The model under review builds one solid part; all positions refer to its coordinate system, in mm. A direction names the side the tool comes from. Give positions to 0.01 mm unless a question says otherwise; leave off trailing zeros. Loops run counter-clockwise (first coordinate to the right, second up) from the corner with the lowest first, then second, coordinate; pieces in that order, holes last. Notation, with made-up numbers: (1.5, 32) - (45.5, 32) arc R26 ccw to (45.5, 65) - close; hole circle Ø6 at (21.25, 42). An arc over 180 degrees is marked (long way). Return JSON: item names as keys, results as strings. Group by question number.
from build123d import *

# Parameters (mm, degrees)
F0_W         = 2.75
F0_H         = 20
F1_DEPTH     = 16
F2_W         = 5.15
F2_H         = 10.3
F3_DEPTH     = 2.75
F4_DEPTH     = 15
F5_T1_DEPTH  = 13.2999992773
F5_T3_DEPTH  = 13.2999992773
F5_T9_DEPTH  = 21.6634917276
F5_T14_DEPTH = 25.0997612432
F5_T22_DEPTH = 21.6634917276
F5_T27_DEPTH = 25.0997612432
F5_T35_DEPTH = 22.0158699277
F5_T40_DEPTH = 25.0997612432
F5_T48_DEPTH = 25.0997612432
F5_T53_DEPTH = 22.0158699277
F6_R         = 5


# Not quite as in the source:
# - a fillet or chamfer that OpenCascade refuses, or shapes differently, is made with other operations: its cross-section is extruded or revolved along the edge and cut away or added
# - a feature names something its author has since deleted; it is built from what else it names


with BuildPart() as f1:
    # F0 (on Top) → F1 (new body)
    with BuildSketch(Plane.XY):
        Rectangle(F0_W, F0_H)
    extrude(amount=F1_DEPTH)

    # F2 (on face) → F3 (join)
    with BuildSketch(Plane.YZ.offset(1.375)):
        Polygon((0, 16), (-10, 16), (-10, 0), (0, 0), (0, 1.4159553841), (-6.6499996386, 1.4159553841), (-6.6499996386, 14.7159546614), (0, 14.7159546614), align=None)
        Polygon((10, 16), (0, 16), (0, 14.7159546614), (6.6499996386, 14.7159546614), (6.6499996386, 1.4159553841), (0, 1.4159553841), (0, 0), (10, 0), align=None)
        with Locations((-2.575, 8.0659550227)):
            Rectangle(F2_W, F2_H)
        with Locations((2.575, 8.0659550227)):
            Rectangle(F2_W, F2_H)
        Polygon((0, 13.2159550227), (0, 14.7159546614), (-6.6499996386, 14.7159546614), (-6.6499996386, 1.4159553841), (0, 1.4159553841), (0, 2.9159550227), (-5.15, 2.9159550227), (-5.15, 13.2159550227), align=None)
        Polygon((6.6499996386, 14.7159546614), (0, 14.7159546614), (0, 13.2159550227), (5.15, 13.2159550227), (5.15, 2.9159550227), (0, 2.9159550227), (0, 1.4159553841), (6.6499996386, 1.4159553841), align=None)
    extrude(amount=-F3_DEPTH)

    # F2 (on face) → F4 (join)
    with BuildSketch(Plane.YZ.offset(1.375)):
        Polygon((0, 13.2159550227), (0, 14.7159546614), (-6.6499996386, 14.7159546614), (-6.6499996386, 1.4159553841), (0, 1.4159553841), (0, 2.9159550227), (-5.15, 2.9159550227), (-5.15, 13.2159550227), align=None)
        Polygon((6.6499996386, 14.7159546614), (0, 14.7159546614), (0, 13.2159550227), (5.15, 13.2159550227), (5.15, 2.9159550227), (0, 2.9159550227), (0, 1.4159553841), (6.6499996386, 1.4159553841), align=None)
    extrude(amount=F4_DEPTH)

    # F5: fillet of radius 5 on 6 edges, made by hand

    # F5_s2 → F5_t1 (join)
    with BuildSketch(Plane.XZ.offset(-6.6499996386)):
        with BuildLine():
            ThreePointArc((1.375, 16), (2.9287180617, 15.0479907955), (4.7203969801, 14.7159546614))
            Line((4.7203969801, 14.7159546614), (1.375, 14.7159546614))
            Line((1.375, 14.7159546614), (1.375, 16))
        make_face()
        with BuildLine():
            ThreePointArc((1.375, 0), (2.9798891295, 1.0484613517), (4.8613482602, 1.4159553841))
            Line((4.8613482602, 1.4159553841), (1.375, 1.4159553841))
            Line((1.375, 1.4159553841), (1.375, 0))
        make_face()
    extrude(amount=F5_T1_DEPTH)

    # F5_s4 → F5_t3 (join)
    with BuildSketch(Plane.XY.offset(1.4159553841)):
        with BuildLine():
            ThreePointArc((1.375, -10), (3.2009454046, -7.5726231419), (6.0949047864, -6.6499996386))
            Line((6.0949047864, -6.6499996386), (1.375, -6.6499996386))
            Line((1.375, -6.6499996386), (1.375, -10))
        make_face()
        with BuildLine():
            ThreePointArc((1.375, 10), (3.2009454046, 7.5726231419), (6.0949047864, 6.6499996386))
            Line((6.0949047864, 6.6499996386), (1.375, 6.6499996386))
            Line((1.375, 6.6499996386), (1.375, 10))
        make_face()
    extrude(amount=F5_T3_DEPTH)


with BuildPart() as f5_tool7:
    # F5_s8 → F5_t9 (new body)
    with BuildSketch(Plane.XZ.offset(-15.013492089)):
        with BuildLine():
            ThreePointArc((1.375, 16), (2.9287180617, 15.0479907955), (4.7203969801, 14.7159546614))
            Line((4.7203969801, 14.7159546614), (1.375, 14.7159546614))
            Line((1.375, 14.7159546614), (1.375, 16))
        make_face()
    extrude(amount=F5_T9_DEPTH)

    split(bisect_by=Plane.XZ.offset(-10), keep=Keep.TOP)

    split(bisect_by=Plane.XZ.offset(-6.6499996386), keep=Keep.BOTTOM)


with BuildPart() as f5_tool12:
    # F5_s13 → F5_t14 (new body)
    with BuildSketch(Plane.XY.offset(1.4159553841)):
        with BuildLine():
            ThreePointArc((1.375, 10), (3.2009454046, 7.5726231419), (6.0949047864, 6.6499996386))
            Line((6.0949047864, 6.6499996386), (1.375, 6.6499996386))
            Line((1.375, 6.6499996386), (1.375, 10))
        make_face()
    extrude(amount=F5_T14_DEPTH)

    split(bisect_by=Plane.XY.offset(16), keep=Keep.BOTTOM)

    split(bisect_by=Plane.XY.offset(14.7159546614), keep=Keep.TOP)


with BuildPart() as f5_tool7_1:
    add(f5_tool7.part)

    # F5_t17: intersect F5_tool12
    add(f5_tool12.part, mode=Mode.INTERSECT)


with BuildPart() as f1_1:
    add(f1.part)

    # F5_t5: union F5_tool7
    add(f5_tool7_1.part)


with BuildPart() as f5_tool20:
    # F5_s21 → F5_t22 (new body)
    with BuildSketch(Plane.XZ.offset(-6.6499996386)):
        with BuildLine():
            ThreePointArc((1.375, 16), (2.9287180617, 15.0479907955), (4.7203969801, 14.7159546614))
            Line((4.7203969801, 14.7159546614), (1.375, 14.7159546614))
            Line((1.375, 14.7159546614), (1.375, 16))
        make_face()
    extrude(amount=F5_T22_DEPTH)

    split(bisect_by=Plane.XZ.offset(10), keep=Keep.BOTTOM)

    split(bisect_by=Plane.XZ.offset(6.6499996386), keep=Keep.TOP)


with BuildPart() as f5_tool25:
    # F5_s26 → F5_t27 (new body)
    with BuildSketch(Plane.XY.offset(26.5157166273)):
        with BuildLine():
            ThreePointArc((1.375, -10), (3.2009454046, -7.5726231419), (6.0949047864, -6.6499996386))
            Line((6.0949047864, -6.6499996386), (1.375, -6.6499996386))
            Line((1.375, -6.6499996386), (1.375, -10))
        make_face()
    extrude(amount=-F5_T27_DEPTH)

    split(bisect_by=Plane.XY.offset(16), keep=Keep.BOTTOM)

    split(bisect_by=Plane.XY.offset(14.7159546614), keep=Keep.TOP)


with BuildPart() as f5_tool20_1:
    add(f5_tool20.part)

    # F5_t30: intersect F5_tool25
    add(f5_tool25.part, mode=Mode.INTERSECT)


with BuildPart() as f1_2:
    add(f1_1.part)

    # F5_t18: union F5_tool20
    add(f5_tool20_1.part)


with BuildPart() as f5_tool33:
    # F5_s34 → F5_t35 (new body)
    with BuildSketch(Plane.XZ.offset(15.365870289)):
        with BuildLine():
            ThreePointArc((1.375, 0), (2.9798891295, 1.0484613517), (4.8613482602, 1.4159553841))
            Line((4.8613482602, 1.4159553841), (1.375, 1.4159553841))
            Line((1.375, 1.4159553841), (1.375, 0))
        make_face()
    extrude(amount=-F5_T35_DEPTH)

    split(bisect_by=Plane.XZ.offset(10), keep=Keep.BOTTOM)

    split(bisect_by=Plane.XZ.offset(6.6499996386), keep=Keep.TOP)


with BuildPart() as f5_tool38:
    # F5_s39 → F5_t40 (new body)
    with BuildSketch(Plane.XY.offset(14.7159546614)):
        with BuildLine():
            ThreePointArc((1.375, -10), (3.2009454046, -7.5726231419), (6.0949047864, -6.6499996386))
            Line((6.0949047864, -6.6499996386), (1.375, -6.6499996386))
            Line((1.375, -6.6499996386), (1.375, -10))
        make_face()
    extrude(amount=-F5_T40_DEPTH)

    split(bisect_by=Plane.XY, keep=Keep.TOP)

    split(bisect_by=Plane.XY.offset(1.4159553841), keep=Keep.BOTTOM)


with BuildPart() as f5_tool33_1:
    add(f5_tool33.part)

    # F5_t43: intersect F5_tool38
    add(f5_tool38.part, mode=Mode.INTERSECT)


with BuildPart() as f1_3:
    add(f1_2.part)

    # F5_t31: union F5_tool33
    add(f5_tool33_1.part)


with BuildPart() as f5_tool46:
    # F5_s47 → F5_t48 (new body)
    with BuildSketch(Plane.XY.offset(-10.3838065819)):
        with BuildLine():
            ThreePointArc((1.375, 10), (3.2009454046, 7.5726231419), (6.0949047864, 6.6499996386))
            Line((6.0949047864, 6.6499996386), (1.375, 6.6499996386))
            Line((1.375, 6.6499996386), (1.375, 10))
        make_face()
    extrude(amount=F5_T48_DEPTH)

    split(bisect_by=Plane.XY, keep=Keep.TOP)

    split(bisect_by=Plane.XY.offset(1.4159553841), keep=Keep.BOTTOM)


with BuildPart() as f5_tool51:
    # F5_s52 → F5_t53 (new body)
    with BuildSketch(Plane.XZ.offset(6.6499996386)):
        with BuildLine():
            ThreePointArc((1.375, 0), (2.9798891295, 1.0484613517), (4.8613482602, 1.4159553841))
            Line((4.8613482602, 1.4159553841), (1.375, 1.4159553841))
            Line((1.375, 1.4159553841), (1.375, 0))
        make_face()
    extrude(amount=-F5_T53_DEPTH)

    split(bisect_by=Plane.XZ.offset(-10), keep=Keep.TOP)

    split(bisect_by=Plane.XZ.offset(-6.6499996386), keep=Keep.BOTTOM)


with BuildPart() as f5_tool46_1:
    add(f5_tool46.part)

    # F5_t56: intersect F5_tool51
    add(f5_tool51.part, mode=Mode.INTERSECT)


with BuildPart() as f1_4:
    add(f1_3.part)

    # F5_t44: union F5_tool46
    add(f5_tool46_1.part)

    # F6
    f6_edges = [f1_4.edges().sort_by_distance(p)[0] for p in [
        (0, -10, 0),
        (0, -10, 16),
        (0, 10, 16),
        (0, 10, 0),
    ]]
    fillet(f6_edges, radius=F6_R)


solid = f1_4.part
Item 1: Tool access review of faces 1 (the face through (1.375, 0, 8)), 2 (the face through (16.375, 6, 8)), 3 (the face through (11, 6.65, 8)), 4 (the face through (11, 0, 1.416)): name each direction out of +Z, -Z, +X, -X, +Y, -Y from which nothing blocks a thin tool from reaching the whole face with its end or side.
Item 2: Take a section at A-A (x = 13.75). State the section outline as (y, z) points.
Item 3: Take a section at B-B (y = -3.5). State the section outline as (x, z) points (3 decimals).
Item 4: Take a section at C-C (z = 10.75). State the section outline as (x, y) points (3 decimals).
Item 5: Mouldability with a two-part tool opening along Z and no side actions: class faces 5 (the face through (0, 8, 1)), 6 (the face through (9, 0, 13.216)), 7 (the face through (0, -10, 8)) as +Z half, -Z half, draft (parallel to the pull), parting line (faces both ways), or undercut.
Item 6: For P1, Ø2, axis at x = 14.5, z = 10, coming from the +Y side; P2, Ø1.5, axis at x = 8, z = 12.5, coming from the -Y side; P3, Ø2, axis at x = 7, z = 9.5, coming from the +Y side, all flat-tipped, find the tip position at first contact; note any pin that passes through.
Item 7: For L1, parallel to Z at x = 9.75, y = 3.5; L2, parallel to Y at x = 9, z = 11.5; L3, parallel to Y at x = 10, z = 2, list the stretches that pass through material, from the lowest coordinate up. Write a range as from..to.
Item 8: Take a section at D-D (x = 4.25). State the section outline as (y, z) points, then the cut area to 3 significant figures.
Check sheet entries:
{
 "1": {"face 1": "+X", "face 2": "+Z, -Z, +X, +Y, -Y", "face 3": "+Z, -Z, +X, +Y", "face 4": "-Z, +X, +Y, -Y"},
 "2": {"outline": "(-6.65, 1.42) - (6.65, 1.42) - (6.65, 14.72) - (-6.65, 14.72) - close; hole (-5.15, 2.92) - (5.15, 2.92) - (5.15, 13.22) - (-5.15, 13.22) - close"},
 "3": {"outline": "(-1.375, 0) - (1.375, 0) arc R5 cw to (4.861, 1.416) - (16.375, 1.416) - (16.375, 2.916) - (1.375, 2.916) - (1.375, 13.216) - (16.375, 13.216) - (16.375, 14.716) - (4.72, 14.716) arc R5 cw to (1.375, 16) - (-1.375, 16) - close"},
 "4": {"outline": "(-1.375, -10) - (1.375, -10) arc R5 cw to (6.095, -6.65) - (16.375, -6.65) - (16.375, -5.15) - (1.375, -5.15) - (1.375, 5.15) - (16.375, 5.15) - (16.375, 6.65) - (6.095, 6.65) arc R5 cw to (1.375, 10) - (-1.375, 10) - close"},
 "5": {"face 5": "-Z half", "face 6": "undercut", "face 7": "draft"},
 "6": {"P1": "stops at y = 6.65", "P2": "stops at y = -6.65", "P3": "stops at y = 6.65"},
 "7": {"L1": "z = 1.42..2.92, 13.22..14.72", "L2": "y = -6.65..-5.15, 5.15..6.65", "L3": "y = -6.65..6.65"},
 "8": {"outline": "(-7, 1.38) - (7, 1.38) - (7, 14.74) - (-7, 14.74) - close; hole (-5.15, 2.92) - (5.15, 2.92) - (5.15, 13.22) - (-5.15, 13.22) - close", "area": "81.0 mm^2"}
}
